Here's how the part is built. I have some questions about the finished solid (model axes, mm). Face numbers are marked on the shaded views. Round coordinates to 2 decimals unless told otherwise and drop trailing zeros. Write each loop counter-clockwise with the first axis right and the second up, starting at its lowest first coordinate (ties: lowest second). Pieces come first, ordered by that corner, then holes. Notation, with made-up numbers: (38.5, 38) - (89.5, 38) arc R17 cw to (89.5, 69) - close; hole circle Ø7 at (5.5, 19.5). An arc over 180 degrees is marked (long way). Write item = value, one per line. Start each with the question number.
Item 1: If we section it at B-B (y = 0.9): Please give me the cut outline in (x, z).
Item 2: Thinking about a two-plate mould opening in Z: for the marked faces 1, 2, 3 and 4, which applies, pulls with the +Z half, pulls with the -Z half, needs draft (parallel to the pull), parting line crosses it, or undercut?
Item 3: If we section it at C-C (x = 43): Please give me the cut outline in (y, z).
Item 4: If I drill on line 1 along Z through (x, y) = (35, 1); line 2 along X through (y, z) = (-0.45, -0.5); line 3 along Y through (x, z) = (30, 5), over which ranges is the centre line in solid material (lowest first)? Write a range as [from, to].
Item 5: If we section it at D-D (x = 6): Please give me the cut outline in (y, z).
Item 6: If we section it at A-A (z = 0): Please give me the cut outline in (x, y).
Item 7: For P1, Ø4, axis at x = 13, z = 0, coming from the -Y side; P2, Ø1.5, axis at x = 33.5, z = -2, coming from the -Y side, each with a flat end and sliding along its axis, tell me the tip position at first contact or that it passes through.
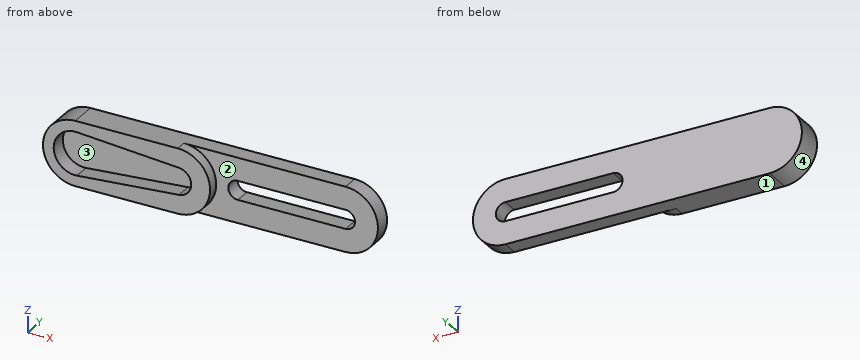
```python
from build123d import *

# Parameters (mm, degrees)
EXTRUDE_1_DEPTH = 3
EXTRUDE_START   = 2
SKETCH_1_4_R    = 4
SKETCH_1_4_R_2  = 2.5
EXTRUDE_2_DEPTH = 2
EXTRUDE_3_DEPTH = 3


with BuildPart() as part:
    # Sketch 1 → Extrude 1 (new body)
    with BuildSketch(Plane(origin=(0, 0, 0), x_dir=(1, 0, 0), z_dir=(0, 1, 0))):
        with BuildLine():
            ThreePointArc((19, -6), (25, 0), (19, 6))
            Line((19, 6), (0, 6))
            ThreePointArc((0, 6), (-6, 0), (0, -6))
            Line((0, -6), (19, -6))
        make_face()
        with BuildLine():
            ThreePointArc((0.315789474, -3.987515142), (-4, 0), (0.315789474, 3.987515142))
            Line((0.315789474, 3.987515142), (19.197368421, 2.492196964))
            ThreePointArc((19.197368421, 2.492196964), (21.5, 0), (19.197368421, -2.492196964))
            Line((19.197368421, -2.492196964), (0.315789474, -3.987515142))
        make_face(mode=Mode.SUBTRACT)
    extrude(amount=-EXTRUDE_1_DEPTH)

    # Sketch 1_4 → Extrude 2 (add)
    with BuildSketch(Plane(origin=(0, 0, 0), x_dir=(1, 0, 0), z_dir=(0, 1, 0)).offset(EXTRUDE_START)):
        Circle(SKETCH_1_4_R)
        with BuildLine():
            ThreePointArc((0.315789474, -3.987515142), (-4, 0), (0.315789474, 3.987515142))
            Line((0.315789474, 3.987515142), (4.773966933, 3.634451777))
            ThreePointArc((4.773966933, 3.634451777), (2.663952828, 5.376184086), (0, 6))
            ThreePointArc((0, 6), (-6, 0), (0, -6))
            ThreePointArc((0, -6), (2.663952828, -5.376184086), (4.773966933, -3.634451777))
            Line((4.773966933, -3.634451777), (0.315789474, -3.987515142))
        make_face()
        with BuildLine():
            Line((4.773966933, 3.634451777), (0.315789474, 3.987515142))
            ThreePointArc((0.315789474, 3.987515142), (2.937954892, 2.71448357), (4, 0))
            ThreePointArc((4, 0), (2.937954892, -2.71448357), (0.315789474, -3.987515142))
            Line((0.315789474, -3.987515142), (4.773966933, -3.634451777))
            ThreePointArc((4.773966933, -3.634451777), (5.685235334, -1.917837115), (6, 0))
            ThreePointArc((6, 0), (5.685235334, 1.917837115), (4.773966933, 3.634451777))
        make_face()
        with BuildLine():
            Line((13.760036579, 2.922804021), (4.773966933, 3.634451777))
            ThreePointArc((4.773966933, 3.634451777), (5.685235334, 1.917837115), (6, 0))
            ThreePointArc((6, 0), (5.685235334, -1.917837115), (4.773966933, -3.634451777))
            Line((4.773966933, -3.634451777), (13.760036579, -2.922804021))
            ThreePointArc((13.760036579, -2.922804021), (13, 0), (13.760036579, 2.922804021))
        make_face()
        with BuildLine():
            ThreePointArc((19, 6), (15.961647167, 5.173819872), (13.760036579, 2.922804021))
            Line((13.760036579, 2.922804021), (19.197368421, 2.492196964))
            ThreePointArc((19.197368421, 2.492196964), (20.836221807, 1.696552231), (21.5, 0))
            ThreePointArc((21.5, 0), (20.836221807, -1.696552231), (19.197368421, -2.492196964))
            Line((19.197368421, -2.492196964), (13.760036579, -2.922804021))
            ThreePointArc((13.760036579, -2.922804021), (15.961647167, -5.173819872), (19, -6))
            ThreePointArc((19, -6), (23.242640687, -4.242640687), (25, 0))
            ThreePointArc((25, 0), (23.242640687, 4.242640687), (19, 6))
        make_face()
        with BuildLine():
            Line((19.197368421, 2.492196964), (13.760036579, 2.922804021))
            ThreePointArc((13.760036579, 2.922804021), (13, 0), (13.760036579, -2.922804021))
            Line((13.760036579, -2.922804021), (19.197368421, -2.492196964))
            ThreePointArc((19.197368421, -2.492196964), (16.5, 0), (19.197368421, 2.492196964))
        make_face()
        with Locations((19, 0)):
            Circle(SKETCH_1_4_R_2)
        with BuildLine():
            ThreePointArc((19, 6), (15.961647167, 5.173819872), (13.760036579, 2.922804021))
            Line((13.760036579, 2.922804021), (19.197368421, 2.492196964))
            ThreePointArc((19.197368421, 2.492196964), (20.836221807, 1.696552231), (21.5, 0))
            ThreePointArc((21.5, 0), (20.836221807, -1.696552231), (19.197368421, -2.492196964))
            Line((19.197368421, -2.492196964), (13.760036579, -2.922804021))
            ThreePointArc((13.760036579, -2.922804021), (15.961647167, -5.173819872), (19, -6))
            ThreePointArc((19, -6), (23.242640687, -4.242640687), (25, 0))
            ThreePointArc((25, 0), (23.242640687, 4.242640687), (19, 6))
        make_face()
        with BuildLine():
            Line((19.197368421, 2.492196964), (13.760036579, 2.922804021))
            ThreePointArc((13.760036579, 2.922804021), (13, 0), (13.760036579, -2.922804021))
            Line((13.760036579, -2.922804021), (19.197368421, -2.492196964))
            ThreePointArc((19.197368421, -2.492196964), (16.5, 0), (19.197368421, 2.492196964))
        make_face()
        with BuildLine():
            ThreePointArc((0, 6), (2.663952828, 5.376184086), (4.773966933, 3.634451777))
            Line((4.773966933, 3.634451777), (13.760036579, 2.922804021))
            ThreePointArc((13.760036579, 2.922804021), (15.961647167, 5.173819872), (19, 6))
            Line((19, 6), (0, 6))
        make_face()
        with BuildLine():
            Line((13.760036579, -2.922804021), (4.773966933, -3.634451777))
            ThreePointArc((4.773966933, -3.634451777), (2.663952828, -5.376184086), (0, -6))
            Line((0, -6), (19, -6))
            ThreePointArc((19, -6), (15.961647167, -5.173819872), (13.760036579, -2.922804021))
        make_face()
        with BuildLine():
            ThreePointArc((0.315789474, -3.987515142), (-4, 0), (0.315789474, 3.987515142))
            Line((0.315789474, 3.987515142), (4.773966933, 3.634451777))
            ThreePointArc((4.773966933, 3.634451777), (2.663952828, 5.376184086), (0, 6))
            ThreePointArc((0, 6), (-6, 0), (0, -6))
            ThreePointArc((0, -6), (2.663952828, -5.376184086), (4.773966933, -3.634451777))
            Line((4.773966933, -3.634451777), (0.315789474, -3.987515142))
        make_face()
        with BuildLine():
            Line((4.773966933, 3.634451777), (0.315789474, 3.987515142))
            ThreePointArc((0.315789474, 3.987515142), (2.937954892, 2.71448357), (4, 0))
            ThreePointArc((4, 0), (2.937954892, -2.71448357), (0.315789474, -3.987515142))
            Line((0.315789474, -3.987515142), (4.773966933, -3.634451777))
            ThreePointArc((4.773966933, -3.634451777), (5.685235334, -1.917837115), (6, 0))
            ThreePointArc((6, 0), (5.685235334, 1.917837115), (4.773966933, 3.634451777))
        make_face()
    extrude(amount=-EXTRUDE_2_DEPTH)

    # Sketch 2 → Extrude 3 (add)
    with BuildSketch(Plane(origin=(0, 2, 0), x_dir=(1, 0, 0), z_dir=(0, 1, 0))):
        with BuildLine():
            ThreePointArc((49, -6), (55, 0), (49, 6))
            Line((49, 6), (19, 6))
            ThreePointArc((19, 6), (25, 0), (19, -6))
            Line((19, -6), (49, -6))
        make_face()
        with BuildLine():
            ThreePointArc((49, 1.75), (50.75, 0), (49, -1.75))
            Line((49, -1.75), (29, -1.75))
            ThreePointArc((29, -1.75), (27.25, 0), (29, 1.75))
            Line((29, 1.75), (49, 1.75))
        make_face(mode=Mode.SUBTRACT)
    extrude(amount=-EXTRUDE_3_DEPTH)


solid = part.part
```
Reply:
q1.outline = (0, -6) - (49, -6) arc R6 ccw to (49, 6) - (0, 6) arc R6 ccw to start; hole (29, -1.75) - (49, -1.75) arc R1.75 ccw to (49, 1.75) - (29, 1.75) arc R1.75 ccw to start
q2.face_1 = pulls with the -Z half
q2.face_2 = needs draft
q2.face_3 = undercut
q2.face_4 = parting line crosses it
q3.outline = (-1, -6) - (2, -6) - (2, -1.75) - (-1, -1.75) - close; (-1, 1.75) - (2, 1.75) - (2, 6) - (-1, 6) - close
q4.line_1 = [-6, -1.75], [1.75, 6]
q4.line_2 = [-5.98, -3.97], [21.45, 27.32], [50.68, 54.98]
q4.line_3 = [-1, 2]
q5.outline = (-3, -6) - (2, -6) - (2, 6) - (-3, 6) - (-3, 3.54) - (0, 3.54) - (0, -3.54) - (-3, -3.54) - close
q6.outline = (-6, -3) - (-4, -3) - (-4, 0) - (21.5, 0) - (21.5, -3) - (25, -3) - (25, -1) - (27.25, -1) - (27.25, 2) - (-6, 2) - close; (50.75, -1) - (55, -1) - (55, 2) - (50.75, 2) - close
q7.P1 = 0
q7.P2 = -1
